```python
from build123d import *

# Parameters (mm, degrees)
SKETCH2_R           = 25
SKETCH2_R_2         = 24
BOSS_EXTRUDE1_DEPTH = 20
CUT_EXTRUDE1_DEPTH  = 21
SKETCH4_W           = 1.280900959
SKETCH4_H           = 0.727497166
CUT_EXTRUDE2_DEPTH  = 21
SKETCH5_W           = 1.000282178
SKETCH5_H           = 20
BOSS_EXTRUDE2_DEPTH = 25
SKETCH6_W           = 15
SKETCH6_H           = 8
CUT_EXTRUDE3_DEPTH  = 38.481628733
SKETCH7_W           = 17
SKETCH7_H           = 10
SKETCH7_W_2         = 15
SKETCH7_H_2         = 8
BOSS_EXTRUDE3_DEPTH = 10


with BuildPart() as part:
    # Sketch2 → Boss-Extrude1 (new body)
    with BuildSketch(Plane.XY):
        Circle(SKETCH2_R)
        Circle(SKETCH2_R_2, mode=Mode.SUBTRACT)
    extrude(amount=BOSS_EXTRUDE1_DEPTH)

    # Sketch3 → Cut-Extrude1 (cut, through all)
    with BuildSketch(Plane.XY.offset(20)):
        Polygon((-12.48839905, 21.657328764), (25, 0), (47.90060784, -51.20755357), (-94.197848054, -17.737254368), align=None)
    extrude(amount=-CUT_EXTRUDE1_DEPTH, mode=Mode.SUBTRACT)

    # Sketch4 → Cut-Extrude2 (cut, through all)
    with BuildSketch(Plane.XY.offset(20)):
        with Locations((24.633397985, 0.218033182)):
            Rectangle(SKETCH4_W, SKETCH4_H)
    extrude(amount=-CUT_EXTRUDE2_DEPTH, mode=Mode.SUBTRACT)

    # Sketch5 → Boss-Extrude2 (add)
    with BuildSketch(Plane.XZ.offset(-0.581781765)):
        with Locations((24.493088594, 10)):
            Rectangle(SKETCH5_W, SKETCH5_H)
    extrude(amount=BOSS_EXTRUDE2_DEPTH)

    # Sketch6 → Cut-Extrude3 (cut, through all)
    with BuildSketch(Plane(origin=(24.993229683, 0, 0), x_dir=(0, 0, -1), z_dir=(1, 0, 0))):
        with Locations((-10, -17.418218235)):
            Rectangle(SKETCH6_W, SKETCH6_H)
    extrude(amount=-CUT_EXTRUDE3_DEPTH, mode=Mode.SUBTRACT)

    # Sketch7 → Boss-Extrude3 (add)
    with BuildSketch(Plane(origin=(24.993229683, 0, 0), x_dir=(0, 0, -1), z_dir=(1, 0, 0))):
        with Locations((-10, -17.418218235)):
            Rectangle(SKETCH7_W, SKETCH7_H)
        with Locations((-10, -17.418218235)):
            Rectangle(SKETCH7_W_2, SKETCH7_H_2, mode=Mode.SUBTRACT)
    extrude(amount=BOSS_EXTRUDE3_DEPTH)


solid = part.part
```
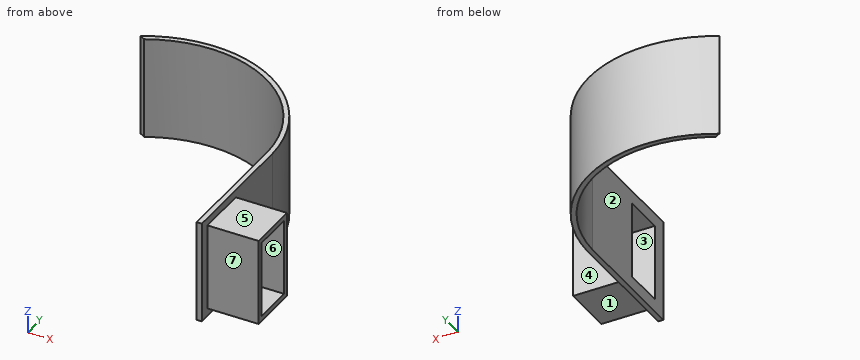
The listing builds one solid part. Answer for the finished solid, in the listing's coordinates (mm). Face numbers are marked on the shaded views. A direction names the side the tool comes from. Coordinates: 2 decimals unless noted, no trailing zeros. Write each loop counter-clockwise with the first axis right and the second up, starting at its lowest first coordinate (ties: lowest second). Pieces come first, ordered by that corner, then holes.
Q1. Section C-C, the plane x = 30 is taken. Write down the section's boundary in (y, z), then the cut area to 3 significant figures.
Returned:
outline: (-22.42, 1.5) - (-12.42, 1.5) - (-12.42, 18.5) - (-22.42, 18.5) - close; hole (-21.42, 2.5) - (-13.42, 2.5) - (-13.42, 17.5) - (-21.42, 17.5) - close
area: 50.0 mm2
Q2. Section D-D, the plane y = -6 is taken. Write down the section's boundary in (x, z), then the cut area to 3 significant figures.
Returned:
outline: (23.99, 0) - (24.99, 0) - (24.99, 20) - (23.99, 20) - close
area: 20.0 mm2
Q3. Which of the six approach directions +Z, -Z, +X, -X, +Y, -Y give full straight-line access (tool end or side, diameter ignored) to the marked faces 4, 5, 6 and 7?
Returned:
face 4: +Z, -Z, +X, +Y
face 5: +Z, +X, +Y, -Y
face 6: +X, -X
face 7: +Z, -Z, +X, -Y
Q4. Section A-A, the plane y = -19.5 is taken. Write down the section's boundary in (x, z).
Returned:
outline: (23.99, 0) - (24.99, 0) - (24.99, 1.5) - (34.99, 1.5) - (34.99, 2.5) - (23.99, 2.5) - close; (23.99, 17.5) - (34.99, 17.5) - (34.99, 18.5) - (24.99, 18.5) - (24.99, 20) - (23.99, 20) - close
Q5. The mould has two halves that part along Z. Classify the marked faces 1, 2 and 3: released by +Z, released by -Z, zero draft, split by the parting line, or undercut.
Returned:
face 1: released by -Z
face 2: zero draft
face 3: undercut
Q6. Find the intervals of material crossed by line 1 along Y through (x, z) = (27, 12.5); line 2 along X through (y, z) = (-9.5, 10.5); line 3 along X through (y, z) = (4, 3.25), in increasing order.
Returned:
line 1: y = -22.42 to -21.42, -13.42 to -12.42
line 2: x = 23.99 to 24.99
line 3: x = 23.66 to 24.68
Q7. Given P1, Ø1, axis at y = -5.5, z = 4.5, coming from the -X side; P2, Ø1, axis at x = 27.5, y = -19, coming from the -Z side; P3, Ø8, axis at x = 29.5, z = 6.5, coming from the +Y side; P4, Ø6.5, axis at x = 28, y = -17.5, coming from the -Z side, each flat-ended and moving along its own axis, determine where each tip first touches the part or whether it passes through.
Returned:
P1: stops at x = 23.99
P2: stops at z = 1.5
P3: stops at y = -12.42
P4: stops at z = 0
Q8. Section B-B, the plane z = 11 is taken. Write down the section's boundary in (x, y), then the cut area to 3 significant figures.
Returned:
outline: (-12.49, 21.66) - (-11.48, 21.08) arc R24 cw to (23.99, 0.58) - (23.99, -13.42) - (34.99, -13.42) - (34.99, -12.42) - (24.99, -12.42) - (24.99, 0.58) arc R25 ccw to start; (23.99, -24.42) - (24.99, -24.42) - (24.99, -22.42) - (34.99, -22.42) - (34.99, -21.42) - (23.99, -21.42) - close
area: 87.4 mm2
